For this review, use the dimensioned drawing (mm, ordinates from the lowest corner) and the shaded views. Give positions to 0.01 mm unless a question says otherwise; leave off trailing zeros. Order: outer loops, then holes, each group sorted by start corner. A loop starts at its lowest first (then second) coordinate and runs counter-clockwise, first axis right, second up. Notation, with made-up numbers: (30, 45.5) - (34, 45.5) arc R20 ccw to (34, 65.5) - close; hole circle Ø1 at (-17.75, -4.5). An arc over 180 degrees is marked (long way). One line per item, written item: value.
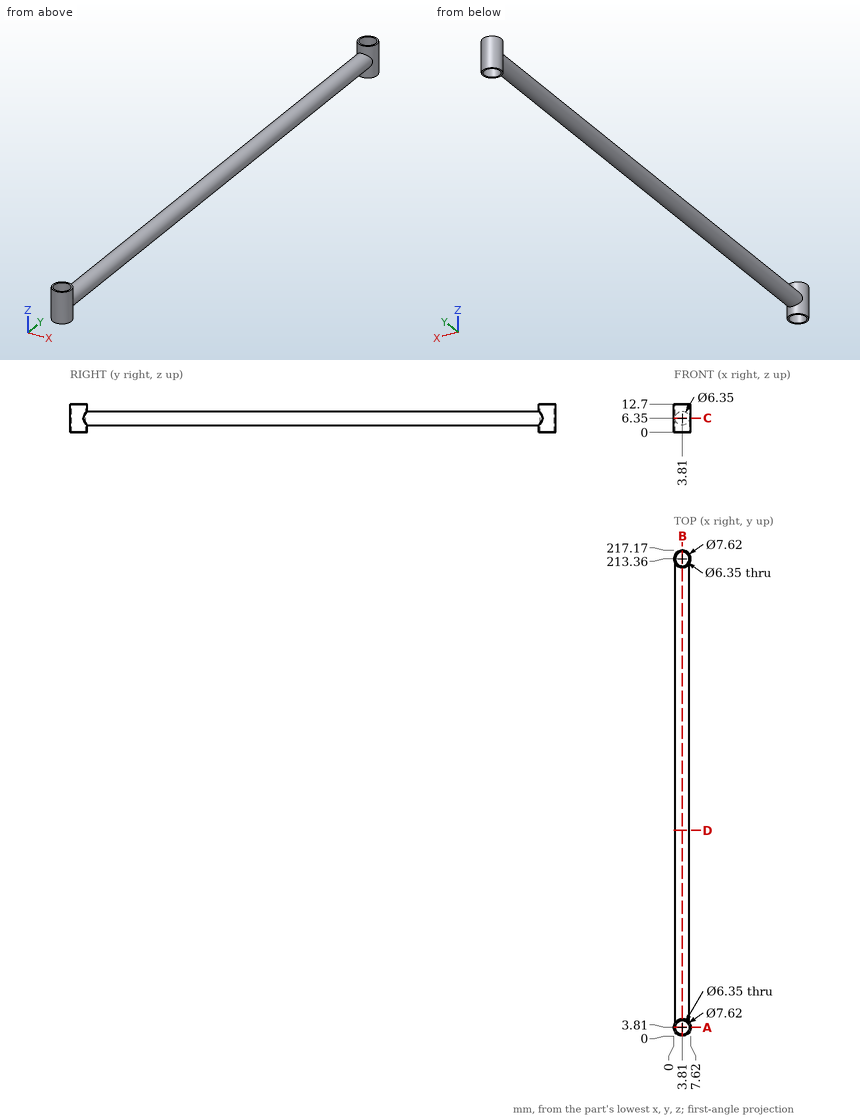
(1) Take a section at D-D (y = 92). Write out the cut boundary in (x, z) (3 decimals), then the cut area to 3 significant figures.
Answers below:
outline: circle Ø6.35 at (3.81, 6.35)
area: 31.7 mm^2
(2) For P1, Ø1, axis at y = 90, z = 4.5, coming from the +X side; P2, Ø1, axis at y = 104, z = 5.5, coming from the -X side; P3, Ø3, axis at x = 2.5, z = 4, coming from the -Y side; P4, Ø1.5, axis at y = 24, z = 4, coming from the +X side, all flat-tipped, find the tip position at first contact; note any pin that passes through.
Answers below:
P1: stops at x = 6.68
P2: stops at x = 0.65
P3: stops at y = 0
P4: stops at x = 6.55
(3) Take a section at A-A (y = 3.81). Write out the cut boundary in (x, z) (3 decimals).
Answers below:
outline: (0, 0) - (0.635, 0) - (0.635, 12.7) - (0, 12.7) - close; (6.985, 0) - (7.62, 0) - (7.62, 12.7) - (6.985, 12.7) - close
(4) Wall thickness on line 1 (Y direction, x = 3.81, z = 3.5) (3 decimals); line 2 (Y direction, x = 4.25, z = 7.5); line 3 (Y direction, x = 3.5, z = 2.5): over which ranges is each line inside the solid? List them lowest first. Write a range as from..to.
Answers below:
line 1: y = 0..0.635, 6.985..210.185, 216.535..217.17
line 2: y = 0.03..0.67, 6.95..210.22, 216.5..217.14
line 3: y = 0.01..0.65, 6.97..7.61, 209.56..210.2, 216.52..217.16
(5) Take a section at C-C (z = 6.35). Write out the cut boundary in (x, y) (3 decimals), then the cut area to 3 significant figures.
Answers below:
outline: (0.635, 5.916) arc R3.81 ccw (long way) to (6.985, 5.916) - (6.985, 211.254) arc R3.81 ccw (long way) to (0.635, 211.254) - close; hole circle Ø6.35 at (3.81, 3.81); hole circle Ø6.35 at (3.81, 213.36)
area: 1,320 mm^2
(6) Take a section at B-B (x = 3.81). Write out the cut boundary in (y, z) (3 decimals), then the cut area to 3 significant figures.
Answers below:
outline: (0, 0) - (0.635, 0) - (0.635, 12.7) - (0, 12.7) - close; (6.985, 0) - (7.62, 0) - (7.62, 3.175) - (209.55, 3.175) - (209.55, 0) - (210.185, 0) - (210.185, 12.7) - (209.55, 12.7) - (209.55, 9.525) - (7.62, 9.525) - (7.62, 12.7) - (6.985, 12.7) - close; (216.535, 0) - (217.17, 0) - (217.17, 12.7) - (216.535, 12.7) - close
area: 1,310 mm^2
